from build123d import *

# Parameters (mm, degrees)
SKETCH_1_R               = 19.75
SKETCH_1_R_2             = 15.75
EXTRUDE_1_DEPTH          = 4
SKETCH_2_R               = 19.75
EXTRUDE_2_DEPTH          = 2
SKETCH_3_R               = 16.5
CUT_EXTRUDE_1_DEPTH      = 4
EXTRUDE_3_DEPTH          = 4
PATTERN_CIRCULAR_1_COUNT = 3
CHAMFER_1_SIZE           = 1
CHAMFER_1_SIZE2          = 1.732050808


with BuildPart() as part:
    # 草图1 → 凸台-拉伸1 (new body)
    with BuildSketch(Plane(origin=(0, 0, 0), x_dir=(1, 0, 0), z_dir=(0, 1, 0))):
        with Locations(Location((0, 0, 0), (0, 0, 270))):
            Circle(SKETCH_1_R)
        with Locations(Location((0, 0, 0), (0, 0, 270))):
            Circle(SKETCH_1_R_2, mode=Mode.SUBTRACT)
    extrude(amount=EXTRUDE_1_DEPTH)

    # 草图2 → 凸台-拉伸2 (add)
    with BuildSketch(Plane(origin=(0, 4, 0), x_dir=(1, 0, 0), z_dir=(0, 1, 0))):
        with Locations(Location((0, 0, 0), (0, 0, 270))):
            Circle(SKETCH_2_R)
    extrude(amount=EXTRUDE_2_DEPTH)

    # 草图3 → 切除-拉伸1 (cut)
    with BuildSketch(Plane.XZ.offset(-4)):
        with Locations(Location((0, 0, 0), (0, 0, 90))):
            Circle(SKETCH_3_R)
    extrude(amount=CUT_EXTRUDE_1_DEPTH, mode=Mode.SUBTRACT)

    # 草图4 → 凸台-拉伸3 (add)
    with BuildSketch(Plane.XZ.offset(-4)):
        with BuildLine():
            ThreePointArc((15.727247344, -4.990359803), (15.284037386, -4.638108653), (15.213331764, -4.07639996))
            ThreePointArc((15.213331764, -4.07639996), (15.75, 0), (15.213331764, 4.07639996))
            ThreePointArc((15.213331764, 4.07639996), (15.284037386, 4.638108653), (15.727247344, 4.990359803))
            ThreePointArc((15.727247344, 4.990359803), (16.5, 0), (15.727247344, -4.990359803))
        make_face()
    extrude_3 = extrude(amount=EXTRUDE_3_DEPTH)

    # 阵列(圆周)1: 凸台-拉伸3 ×3 about axis
    pattern_circular_1_axis = Axis((0, 0, 0), (0, 1, 0))
    for i in range(1, PATTERN_CIRCULAR_1_COUNT):
        add(extrude_3.rotate(pattern_circular_1_axis, i * 360 / PATTERN_CIRCULAR_1_COUNT))

    # 倒角1
    chamfer_1_edges = [part.edges().sort_by_distance(p)[0] for p in [
        (0, 6, -19.75),
    ]]
    chamfer_1_side = [part.faces().sort_by_distance(p)[0] for p in [
        (0, 6, 0),
    ]]
    chamfer(chamfer_1_edges, length=CHAMFER_1_SIZE, length2=CHAMFER_1_SIZE2, reference=chamfer_1_side[0])


solid = part.part
The listing builds one solid part. Answer for the finished solid, in the listing's coordinates (mm). A direction names the side the tool comes from. Coordinates: 2 decimals unless noted, no trailing zeros. Write each loop counter-clockwise with the first axis right and the second up, starting at its lowest first coordinate (ties: lowest second). Pieces come first, ordered by that corner, then holes. Notation, with made-up numbers: M 26.25,81.25 L 31.25,81.25 A18 cw 31.25,92.25 Z; hole C 65,-9 d3. An arc over 180 degrees is marked long. Use one line per item in the form item = value.
Item 1: Find section B-B, the plane x = 0. Give the vertices of the cut face in (y, z).
Model answer:
outline = M 0,-19.75 L 4.27,-19.75 L 6,-18.75 L 6,18.75 L 4.27,19.75 L 0,19.75 L 0,16.5 L 4,16.5 L 4,-16.5 L 0,-16.5 Z
Item 2: Find the intervals of material crossed by probe 1 along Y at (x, z) = (-9, -8); probe 2 along Z at (x, y) = (7, 2.85); probe 3 along Z at (x, y) = (-13.5, 3), in increasing order.
Model answer:
probe_1 = 4 to 6
probe_2 = -18.47 to -14.94, 14.94 to 18.47
probe_3 = -14.42 to -9.49, 9.49 to 14.42
Item 3: Find section A-A, the plane y = 2.75. Give the vertices of the cut face in (x, z).
Model answer:
outline = C 0,0 d39.5; hole M -12.19,-11.13 A0.75 cw -11.14,-11.14 A15.75 ccw -4.08,-15.21 A0.75 cw -3.54,-16.12 A16.5 ccw 15.73,-4.99 A0.75 cw 15.21,-4.08 A15.75 ccw 15.21,4.08 A0.75 cw 15.73,4.99 A16.5 ccw -3.54,16.12 A0.75 cw -4.08,15.21 A15.75 ccw -11.14,11.14 A0.75 cw -12.19,11.13 A16.5 ccw Z
Item 4: Find section C-C, the plane z = 0. Give the vertices of the cut face in (x, y).
Model answer:
outline = M -19.75,0 L -16.5,0 L -16.5,4 L 15.75,4 L 15.75,0 L 19.75,0 L 19.75,4.27 L 18.75,6 L -18.75,6 L -19.75,4.27 Z
Item 5: Given P1, Ø1.5, axis at x = 12, y = 3, coming from the -Z side; P2, Ø1.5, axis at x = 9, z = 11, coming from the -Y side; P3, Ø12, axis at x = 1.5, z = 14.5, coming from the -Y side; P4, Ø3, axis at y = 2.5, z = -11.5, coming from the +X side, each flat-ended and moving along its own axis, determine where each tip first touches the part or whether it passes through.
Model answer:
P1 = -16.23
P2 = 4
P3 = 0
P4 = 17.03
Item 6: The mould has two halves that part along X. Classify faces 1 (the face through (15.29, 2.03, -4.65)), 2 (the face through (15.75, 2.03, -0.06)), 3 (the face through (5.93, 2.1, 18.84)), 4 (the face through (0, 6, 0)): released by +X, released by -X, zero draft, split by the parting line, or undercut.
Model answer:
face_1 = undercut
face_2 = undercut
face_3 = split by the parting line
face_4 = zero draft
Item 7: For faces 5 (the face through (-1, 4, 0)), 6 (the face through (16, 0, -2)), determine the directions among +Z, -Z, +X, -X, +Y, -Y from which every point of the face is accessible in a straight line to the end or side of a thin tool.
Model answer:
face_5 = -Y
face_6 = +Z, -Z, +X, -X, -Y
Item 8: Find section D-D, the plane y = 5.1. Give the vertices of the cut face in (x, z).
Model answer:
outline = C 0,0 d38.54
